from build123d import *

# Parameters (mm, degrees)
RESSALTO_EXTRUS_O1_DEPTH = 10
RESSALTO_EXTRUS_O2_DEPTH = 10
CORTE_EXTRUS_O1_START    = 21
ESBO_O4_R                = 6
ESBO_O4_R_2              = 2.5
CORTE_EXTRUS_O1_DEPTH    = 21
RESSALTO_EXTRUS_O3_DEPTH = 2.5


with BuildPart() as part:
    # Esboço1 → Ressalto-extrusão1 (new, symmetric)
    with BuildSketch(Plane(origin=(0, 0, 0), x_dir=(1, 0, 0), z_dir=(0, 1, 0))):
        with BuildLine():
            Line((21, 16), (21, 0))
            Line((21, 0), (24, 0))
            Line((24, 0), (24, 17.242640687))
            Line((24, 17.242640687), (17.242640687, 24))
            Line((17.242640687, 24), (11, 24))
            Line((11, 24), (11, 29))
            ThreePointArc((11, 29), (10.707106781, 29.707106781), (10, 30))
            Line((10, 30), (0, 30))
            Line((0, 30), (-10, 30))
            ThreePointArc((-10, 30), (-10.707106781, 29.707106781), (-11, 29))
            Line((-11, 29), (-11, 24))
            Line((-11, 24), (-17.242640687, 24))
            Line((-17.242640687, 24), (-24, 17.242640687))
            Line((-24, 17.242640687), (-24, 0))
            Line((-24, 0), (-21, 0))
            Line((-21, 0), (-21, 16))
            Line((-21, 16), (-16, 21))
            Line((-16, 21), (-8, 21))
            Line((-8, 21), (-8, 26))
            ThreePointArc((-8, 26), (-7.707106781, 26.707106781), (-7, 27))
            Line((-7, 27), (0, 27))
            Line((0, 27), (7, 27))
            ThreePointArc((7, 27), (7.707106781, 26.707106781), (8, 26))
            Line((8, 26), (8, 21))
            Line((8, 21), (16, 21))
            Line((16, 21), (21, 16))
        make_face()
        Polygon((0, -21), (0, -24), (17.242640687, -24), (24, -17.242640687), (24, 0), (21, 0), (21, -16), (16, -21), align=None)
        Polygon((-17.242640687, -24), (0, -24), (0, -21), (-16, -21), (-21, -16), (-21, 0), (-24, 0), (-24, -17.242640687), align=None)
    extrude(amount=RESSALTO_EXTRUS_O1_DEPTH, both=True)

    # Esboço2 → Ressalto-extrusão2 (add, symmetric)
    with BuildSketch(Plane.XY):
        with BuildLine():
            Line((-24, 0), (-24, 4.5))
            Line((-24, 4.5), (-28, 4.5))
            Line((-28, 4.5), (-28, 2.5))
            ThreePointArc((-28, 2.5), (-26.232233047, 1.767766953), (-25.5, 0))
            Line((-25.5, 0), (-24, 0))
        make_face()
        with BuildLine():
            Line((-28, 2.5), (-28, 4.5))
            Line((-28, 4.5), (-32, 2.5))
            Line((-32, 2.5), (-32, 0))
            Line((-32, 0), (-30.5, 0))
            ThreePointArc((-30.5, 0), (-29.767766953, 1.767766953), (-28, 2.5))
        make_face()
        with BuildLine():
            Line((-24, -4.5), (-24, 0))
            Line((-24, 0), (-25.5, 0))
            ThreePointArc((-25.5, 0), (-28, -2.5), (-30.5, 0))
            Line((-30.5, 0), (-32, 0))
            Line((-32, 0), (-32, -2.5))
            Line((-32, -2.5), (-28, -4.5))
            Line((-28, -4.5), (-24, -4.5))
        make_face()
        with BuildLine():
            Line((32, 0), (30.5, 0))
            ThreePointArc((30.5, 0), (28, -2.5), (25.5, 0))
            Line((25.5, 0), (24, 0))
            Line((24, 0), (24, -4.5))
            Line((24, -4.5), (28, -4.5))
            Line((28, -4.5), (32, -2.5))
            Line((32, -2.5), (32, 0))
        make_face()
        with BuildLine():
            Line((24, 0), (25.5, 0))
            ThreePointArc((25.5, 0), (26.232233047, 1.767766953), (28, 2.5))
            Line((28, 2.5), (28, 4.5))
            Line((28, 4.5), (24, 4.5))
            Line((24, 4.5), (24, 0))
        make_face()
        with BuildLine():
            ThreePointArc((28, 2.5), (29.767766953, 1.767766953), (30.5, 0))
            Line((30.5, 0), (32, 0))
            Line((32, 0), (32, 2.5))
            Line((32, 2.5), (28, 4.5))
            Line((28, 4.5), (28, 2.5))
        make_face()
    extrude(amount=RESSALTO_EXTRUS_O2_DEPTH, both=True)

    # Esboço4 → Corte-extrusão1 (cut)
    # profile 1 of 3: a face of its own
    with BuildSketch(Plane.XY.offset(10).offset(CORTE_EXTRUS_O1_START)):
        with BuildLine():
            Line((-24, 4.472135955), (-24, -4.472135955))
            ThreePointArc((-24, -4.472135955), (-22.522774425, -2.449489743), (-22, 0))
            ThreePointArc((-22, 0), (-22.522774425, 2.449489743), (-24, 4.472135955))
        make_face()
    # profile 2 of 3: a face of its own
    with BuildSketch(Plane.XY.offset(10).offset(CORTE_EXTRUS_O1_START)):
        with Locations((28, 0)):
            Circle(ESBO_O4_R)
        with Locations((28, 0)):
            Circle(ESBO_O4_R_2, mode=Mode.SUBTRACT)
    # profile 3 of 3: a face of its own
    with BuildSketch(Plane.XY.offset(10).offset(CORTE_EXTRUS_O1_START)):
        with Locations((28, 0)):
            Circle(ESBO_O4_R_2)
    extrude(amount=-CORTE_EXTRUS_O1_DEPTH, mode=Mode.SUBTRACT)

    # Esboço5 → Ressalto-extrusão3 (add, symmetric)
    # profile 1 of 4: a face of its own
    with BuildSketch(Plane(origin=(0, 0, -10), x_dir=(-1, 0, 0), z_dir=(0, 0, -1))):
        Polygon((-28, 6.736067977), (-22, 3.736067977), (-22, -3.736067977), (-28, -6.736067977), (-34, -3.736067977), (-34, 3.736067977), align=None)
        Polygon((-28, 4.5), (-32, 2.5), (-32, -2.5), (-28, -4.5), (-24, -4.5), (-24, 4.5), align=None, mode=Mode.SUBTRACT)
    # profile 2 of 4: a face of its own
    with BuildSketch(Plane(origin=(0, 0, -10), x_dir=(-1, 0, 0), z_dir=(0, 0, -1))):
        Polygon((-24, 4.5), (-28, 4.5), (-24, 2.5), align=None)
    # profile 3 of 4: a face of its own
    with BuildSketch(Plane(origin=(0, 0, -10), x_dir=(-1, 0, 0), z_dir=(0, 0, -1))):
        Polygon((-24, -2.5), (-28, -4.5), (-24, -4.5), align=None)
    # profile 4 of 4: a face of its own
    with BuildSketch(Plane(origin=(0, 0, -10), x_dir=(-1, 0, 0), z_dir=(0, 0, -1))):
        Polygon((28, 6.736067977), (34, 3.736067977), (34, -3.736067977), (28, -6.736067977), (22, -3.736067977), (22, 3.736067977), align=None)
        Polygon((28, 4.5), (32, 2.5), (32, -2.5), (28, -4.5), (24, -2.5), (24, 2.5), align=None, mode=Mode.SUBTRACT)
    extrude(amount=RESSALTO_EXTRUS_O3_DEPTH, both=True)


solid = part.part
Input: part model. Units: mm. Frame: model coordinates. A direction names the side the tool comes from. Coordinates: 2 decimals unless noted, no trailing zeros. Loops run counter-clockwise (first coordinate to the right, second up) from the corner with the lowest first, then second, coordinate; pieces in that order, holes last. Notation, with made-up numbers: (81.25, 71.25) -> (88.25, 71.25) arc R9 cw to (88.25, 88.25) -> close; hole circle Ø1 at (75.5, -24). An arc over 180 degrees is marked (long way). Write each question's results on one line, items separated by ' | '. Start each with the question number.
Q1. Section B-B, the plane y = 7.75. Return the cut outline in (x, z).
Q2. Section C-C, the plane z = 13.5. Return the cut outline in (x, y).
Q3. Pull-direction query (X, two-part tool) for faces 1 (the flat face through (31.042, 5.215, -9.965)), 2 (the flat face through (-30, -3.5, 1.1)), 3 (the flat face through (12, 0, -21)), 4 (the flat face through (0, 0, 24)); classes: released by +X, released by -X, zero draft, split by the parting line, or undercut.
Q4. Pin query (flat end, axial travel): pin 1 (3 mm diameter, centred on y = 1, z = -21, fed in from -X); pin 2 (11 mm diameter, centred on x = -28, y = 0, fed in from +Z); pin 3 (1.2 mm diameter, centred on x = -25, z = -1.5, fed in from +Y); pin 4 (8 mm diameter, centred on x = -15, z = -16, fed in from -Y). Return the tip coordinate at first contact, or that it passes through.
Q5. Ray query, line 1 (X direction, y = 0, z = -4.5); line 2 (X direction, y = -2.5, z = -12); line 3 (Z direction, x = 12, y = -4.25). Return the intervals inside material, ascending. Write a range as from..to.
Q6. Section D-D, the plane x = -9. Return the cut outline in (y, z).
Q7. Reachability of faces 5 (the flat face through (26, 4.5, 1)), 6 (the flat face through (-12, 0, -21)), 7 (the flat face through (26, -4.5, 1)), 8 (the flat face through (25.97, -5.72, -9.96)) from +Z, -Z, +X, -X, +Y, -Y: full face, straight path, thin tool, end or side. Return the list, or none.
Q8. Section A-A, the plane x = 1. Return the cut outline in (y, z).
Found:
1) outline: (-24, -17.24) -> (-17.24, -24) -> (-11, -24) -> (-11, -29) arc R1 ccw to (-10, -30) -> (10, -30) arc R1 ccw to (11, -29) -> (11, -24) -> (17.24, -24) -> (24, -17.24) -> (24, 17.24) -> (17.24, 24) -> (-17.24, 24) -> (-24, 17.24) -> close; hole (-21, -16) -> (-16, -21) -> (-8, -21) -> (-8, -26) arc R1 ccw to (-7, -27) -> (7, -27) arc R1 ccw to (8, -26) -> (8, -21) -> (16, -21) -> (21, -16) -> (21, 16) -> (16, 21) -> (-16, 21) -> (-21, 16) -> close
2) outline: (-24, -10) -> (-21, -10) -> (-21, 10) -> (-24, 10) -> (-24, 4.47) arc R6 cw to (-24, -4.47) -> close; (21, -10) -> (24, -10) -> (24, -4.47) arc R6 cw to (24, 4.47) -> (24, 10) -> (21, 10) -> close
3) face 1: released by +X | face 2: released by -X | face 3: undercut | face 4: zero draft
4) pin 1: x = -21.74 | pin 2: z = 10 | pin 3: y = 4.5 | pin 4: through
5) line 1: -32..-30.5, -25.5..-21, 21..25.5, 30.5..32 | line 2: -34..-32, -24..-21, 21..24, 32..34 | line 3: -24..-21, 21..24
6) outline: (-10, -30) -> (10, -30) -> (10, -21) -> (-10, -21) -> close; (-10, 21) -> (10, 21) -> (10, 24) -> (-10, 24) -> close
7) face 5: +Z, +X, +Y | face 6: +Y, -Y | face 7: +Z, +X, -Y | face 8: +Z, -Z, -Y
8) outline: (-10, -30) -> (10, -30) -> (10, -27) -> (-10, -27) -> close; (-10, 21) -> (10, 21) -> (10, 24) -> (-10, 24) -> close
